The model under review builds one solid part; all positions refer to its coordinate system, in mm. Face numbers are marked on the shaded views. A direction names the side the tool comes from. Round coordinates to 2 decimals unless told otherwise and drop trailing zeros. Write each loop counter-clockwise with the first axis right and the second up, starting at its lowest first coordinate (ties: lowest second). Pieces come first, ordered by that corner, then holes. Notation, with made-up numbers: (-5, 25) -> (31, 25) arc R10 cw to (31, 31) -> close; hole circle Ø11 at (63.5, 26.25). An arc over 180 degrees is marked (long way). Answer as a JSON object with one key per item and string values. Group by question number.
1) Machinability: for the marked faces 1, 2 and 3, which of the approach directions +Z, -Z, +X, -X, +Y, -Y give a long, thin tool a straight path to every point of the face, cutting with its end or side? Answer none if there is none.
2) Mouldability with a two-part tool opening along Z and no side actions: class the marked faces 4, 5 and 6 as pulls with the +Z half, pulls with the -Z half, needs draft (parallel to the pull), parting line crosses it, or undercut.
3) Insertion check: pin 1 Ø8 at (x, z) = (1.5, 3.5) entering from -Y (3 decimals); pin 2 Ø3 at (y, z) = (5.5, -4.5) entering from -X; pin 3 Ø3 at (x, z) = (2.5, 3) entering from +Y (3 decimals). Each pin has a flat end and moves straight along its axis. Give the tip position at first contact, or say it passes through.
4) To check wall thickness, follow probe 1 along X at (y, z) = (1.75, 2.5); probe 2 along X at (y, z) = (6.7, 0); probe 3 along Y at (x, z) = (6.75, -1). State the ranges of each line that lie inside material, in increasing order. Write a range as [from, to].
5) We need section A-A, the plane y = 2.25. Write out the cut boundary in (x, z), then the cut area to 3 significant figures.
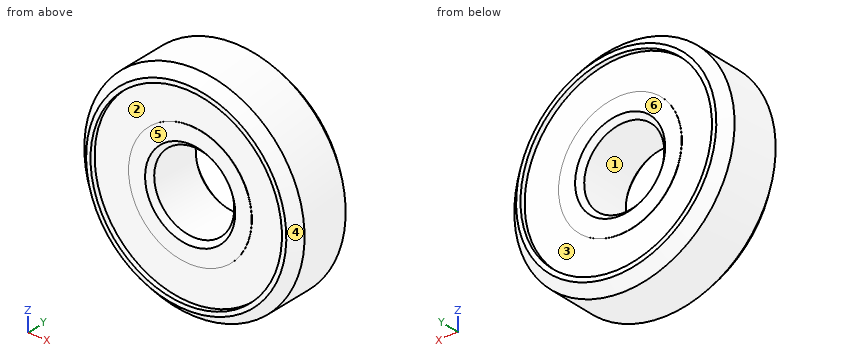
from build123d import *

# Parameters (mm, degrees)
SKETCH1_R                = 11
SKETCH1_R_2              = 4
BOSS_EXTRUDE1_DEPTH      = 7
CHAMFER1_SIZE            = 1
SKETCH2_R                = 9.560499877
CUT_EXTRUDE1_DEPTH       = 0.5
SKETCH3_R                = 6.152500931
SKETCH3_R_2              = 4
BOSS_EXTRUDE2_DEPTH      = 0.025
CHAMFER2_SIZE            = 0.5
CHAMFER2_OF_MIRROR3_SIZE = 0.5


with BuildPart() as part:
    # Sketch1 → Boss-Extrude1 (new body)
    with BuildSketch(Plane(origin=(0, 0, 0), x_dir=(1, 0, 0), z_dir=(0, 1, 0))):
        with Locations(Location((0, 0, 0), (0, 0, 270))):
            Circle(SKETCH1_R)
        with Locations(Location((0, 0, 0), (0, 0, 270))):
            Circle(SKETCH1_R_2, mode=Mode.SUBTRACT)
    extrude(amount=BOSS_EXTRUDE1_DEPTH)

    # Chamfer1
    chamfer1_edges = [part.edges().sort_by_distance(p)[0] for p in [
        (0, 0, -11),
        (0, 7, -11),
    ]]
    chamfer(chamfer1_edges, length=CHAMFER1_SIZE)

    # Sketch2 → Cut-Extrude1 (cut)
    with BuildSketch(Plane(origin=(0, 7, 0), x_dir=(1, 0, 0), z_dir=(0, 1, 0))):
        with Locations(Location((0, 0, 0), (0, 0, 270))):
            Circle(SKETCH2_R)
    cut_extrude1 = extrude(amount=-CUT_EXTRUDE1_DEPTH, mode=Mode.SUBTRACT)

    # Sketch3 → Boss-Extrude2 (add)
    with BuildSketch(Plane(origin=(0, 6.5, 0), x_dir=(1, 0, 0), z_dir=(0, 1, 0))):
        with Locations(Location((0, 0, 0), (0, 0, 270))):
            Circle(SKETCH3_R)
        with Locations(Location((0, 0, 0), (0, 0, 270))):
            Circle(SKETCH3_R_2, mode=Mode.SUBTRACT)
    boss_extrude2 = extrude(amount=BOSS_EXTRUDE2_DEPTH)

    # Chamfer2
    chamfer2_edges = [part.edges().sort_by_distance(p)[0] for p in [
        (0, 6.525, -4),
    ]]
    chamfer(chamfer2_edges, length=CHAMFER2_SIZE)

    # Mirror3: Cut-Extrude1, Boss-Extrude2 across plane
    add(cut_extrude1.mirror(Plane(origin=(0, 3.500000112, 0), x_dir=(0, 0, 1), z_dir=(0, -1, 0))), mode=Mode.SUBTRACT)
    add(boss_extrude2.mirror(Plane(origin=(0, 3.500000112, 0), x_dir=(0, 0, 1), z_dir=(0, -1, 0))))

    # Chamfer2 of Mirror3
    chamfer2_of_mirror3_edges = [part.edges().sort_by_distance(p)[0] for p in [
        (0, 0.475000224, -4),
    ]]
    chamfer(chamfer2_of_mirror3_edges, length=CHAMFER2_OF_MIRROR3_SIZE)


solid = part.part
Here are the results:
{
 "1": {"face 1": "+Y, -Y", "face 2": "-Y", "face 3": "+Y"},
 "2": {"face 4": "parting line crosses it", "face 5": "undercut", "face 6": "undercut"},
 "3": {"pin 1": "stops at y = 0.475", "pin 2": "stops at x = -10.58", "pin 3": "stops at y = 6.525"},
 "4": {"probe 1": "x = [-10.71, -3.12], [3.12, 10.71]", "probe 2": "x = [-10.3, -9.56], [9.56, 10.3]", "probe 3": "y = [0.5, 6.5]"},
 "5": {"outline": "circle Ø22 at (0, 0); hole circle Ø8 at (0, 0)", "area": "330 mm^2"}
}
